```python
from build123d import *

# Parameters (mm, degrees)
F0_R     = 3.1
F0_R_2   = 1.6
F1_DEPTH = 5


with BuildPart() as f1:
    # F0 (on Front) → F1 (new body)
    with BuildSketch(Plane.XZ):
        with BuildLine():
            Line((10.150758, 20), (-10.150758, 20))
            ThreePointArc((-10.150758, 20), (-12.064175, 20.380602), (-13.686292, 21.464466))
            Line((-13.686292, 21.464466), (-61.509049, 69.287223))
            Line((-61.509049, 69.287223), (-67.386104, 73.484299))
            ThreePointArc((-67.386104, 73.484299), (-72.699434, 72.699434), (-73.484299, 67.386104))
            Line((-73.484299, 67.386104), (-69.287223, 61.509049))
            Line((-69.287223, 61.509049), (-21.464466, 13.686292))
            ThreePointArc((-21.464466, 13.686292), (-20.380602, 12.064175), (-20, 10.150758))
            Line((-20, 10.150758), (-20, -10.150758))
            ThreePointArc((-20, -10.150758), (-20.380602, -12.064175), (-21.464466, -13.686292))
            Line((-21.464466, -13.686292), (-69.287223, -61.509049))
            Line((-69.287223, -61.509049), (-73.484299, -67.386104))
            ThreePointArc((-73.484299, -67.386104), (-72.699434, -72.699434), (-67.386104, -73.484299))
            Line((-67.386104, -73.484299), (-61.509049, -69.287223))
            Line((-61.509049, -69.287223), (-13.686292, -21.464466))
            ThreePointArc((-13.686292, -21.464466), (-12.064175, -20.380602), (-10.150758, -20))
            Line((-10.150758, -20), (10.150758, -20))
            ThreePointArc((10.150758, -20), (12.064175, -20.380602), (13.686292, -21.464466))
            Line((13.686292, -21.464466), (61.509049, -69.287223))
            Line((61.509049, -69.287223), (67.386104, -73.484299))
            ThreePointArc((67.386104, -73.484299), (72.699434, -72.699434), (73.484299, -67.386104))
            Line((73.484299, -67.386104), (69.287223, -61.509049))
            Line((69.287223, -61.509049), (21.464466, -13.686292))
            ThreePointArc((21.464466, -13.686292), (20.380602, -12.064175), (20, -10.150758))
            Line((20, -10.150758), (20, 10.150758))
            ThreePointArc((20, 10.150758), (20.380602, 12.064175), (21.464466, 13.686292))
            Line((21.464466, 13.686292), (69.287223, 61.509049))
            Line((69.287223, 61.509049), (73.484299, 67.386104))
            ThreePointArc((73.484299, 67.386104), (72.699434, 72.699434), (67.386104, 73.484299))
            Line((67.386104, 73.484299), (61.509049, 69.287223))
            Line((61.509049, 69.287223), (13.686292, 21.464466))
            ThreePointArc((13.686292, 21.464466), (12.064175, 20.380602), (10.150758, 20))
        make_face()
        with BuildLine():
            ThreePointArc((-62.586144, -64.848885), (-64.848885, -64.848885), (-64.848885, -62.586144))
            Line((-64.848885, -62.586144), (-63.788225, -61.525483))
            ThreePointArc((-63.788225, -61.525483), (-61.525483, -61.525483), (-61.525483, -63.788225))
            Line((-61.525483, -63.788225), (-62.586144, -64.848885))
        make_face(mode=Mode.SUBTRACT)
        with Locations((-57, -57)):
            Circle(F0_R, mode=Mode.SUBTRACT)
        with BuildLine():
            ThreePointArc((-51.413856, -49.151115), (-49.151115, -49.151115), (-49.151115, -51.413856))
            Line((-49.151115, -51.413856), (-50.211775, -52.474517))
            ThreePointArc((-50.211775, -52.474517), (-52.474517, -52.474517), (-52.474517, -50.211775))
            Line((-52.474517, -50.211775), (-51.413856, -49.151115))
        make_face(mode=Mode.SUBTRACT)
        with Locations((-20.584001, -20.584001)):
            Circle(F0_R_2, mode=Mode.SUBTRACT)
        with Locations((-15.5, -15.5)):
            Circle(F0_R_2, mode=Mode.SUBTRACT)
        with BuildLine():
            ThreePointArc((64.848885, -62.586144), (64.848885, -64.848885), (62.586144, -64.848885))
            Line((62.586144, -64.848885), (61.525483, -63.788225))
            ThreePointArc((61.525483, -63.788225), (61.525483, -61.525483), (63.788225, -61.525483))
            Line((63.788225, -61.525483), (64.848885, -62.586144))
        make_face(mode=Mode.SUBTRACT)
        with Locations((57, -57)):
            Circle(F0_R, mode=Mode.SUBTRACT)
        with BuildLine():
            ThreePointArc((49.151115, -51.413856), (49.151115, -49.151115), (51.413856, -49.151115))
            Line((51.413856, -49.151115), (52.474517, -50.211775))
            ThreePointArc((52.474517, -50.211775), (52.474517, -52.474517), (50.211775, -52.474517))
            Line((50.211775, -52.474517), (49.151115, -51.413856))
        make_face(mode=Mode.SUBTRACT)
        with Locations((20.584001, -20.584001)):
            Circle(F0_R_2, mode=Mode.SUBTRACT)
        with Locations((15.5, -15.5)):
            Circle(F0_R_2, mode=Mode.SUBTRACT)
        with BuildLine():
            ThreePointArc((-10.80108, 10.5), (-10.654634, 10.853553), (-10.30108, 11))
            Line((-10.30108, 11), (-8.80108, 11))
            ThreePointArc((-8.80108, 11), (-8.447527, 10.853553), (-8.30108, 10.5))
            Line((-8.30108, 10.5), (-8.30108, -10.5))
            ThreePointArc((-8.30108, -10.5), (-8.447527, -10.853553), (-8.80108, -11))
            Line((-8.80108, -11), (-10.30108, -11))
            ThreePointArc((-10.30108, -11), (-10.654634, -10.853553), (-10.80108, -10.5))
            Line((-10.80108, -10.5), (-10.80108, 10.5))
        make_face(mode=Mode.SUBTRACT)
        with Locations((-15.5, 15.5)):
            Circle(F0_R_2, mode=Mode.SUBTRACT)
        with Locations((-20.584001, 20.584001)):
            Circle(F0_R_2, mode=Mode.SUBTRACT)
        with BuildLine():
            Line((-50.211775, 52.474517), (-49.151115, 51.413856))
            ThreePointArc((-49.151115, 51.413856), (-49.151115, 49.151115), (-51.413856, 49.151115))
            Line((-51.413856, 49.151115), (-52.474517, 50.211775))
            ThreePointArc((-52.474517, 50.211775), (-52.474517, 52.474517), (-50.211775, 52.474517))
        make_face(mode=Mode.SUBTRACT)
        with Locations((-57, 57)):
            Circle(F0_R, mode=Mode.SUBTRACT)
        with BuildLine():
            ThreePointArc((-64.848885, 62.586144), (-64.848885, 64.848885), (-62.586144, 64.848885))
            Line((-62.586144, 64.848885), (-61.525483, 63.788225))
            ThreePointArc((-61.525483, 63.788225), (-61.525483, 61.525483), (-63.788225, 61.525483))
            Line((-63.788225, 61.525483), (-64.848885, 62.586144))
        make_face(mode=Mode.SUBTRACT)
        with BuildLine():
            Line((10.80108, 10.5), (10.80108, -10.5))
            ThreePointArc((10.80108, -10.5), (10.654634, -10.853553), (10.30108, -11))
            Line((10.30108, -11), (8.80108, -11))
            ThreePointArc((8.80108, -11), (8.447527, -10.853553), (8.30108, -10.5))
            Line((8.30108, -10.5), (8.30108, 10.5))
            ThreePointArc((8.30108, 10.5), (8.447527, 10.853553), (8.80108, 11))
            Line((8.80108, 11), (10.30108, 11))
            ThreePointArc((10.30108, 11), (10.654634, 10.853553), (10.80108, 10.5))
        make_face(mode=Mode.SUBTRACT)
        with Locations((15.5, 15.5)):
            Circle(F0_R_2, mode=Mode.SUBTRACT)
        with Locations((20.584001, 20.584001)):
            Circle(F0_R_2, mode=Mode.SUBTRACT)
        with BuildLine():
            Line((52.474517, 50.211775), (51.413856, 49.151115))
            ThreePointArc((51.413856, 49.151115), (49.151115, 49.151115), (49.151115, 51.413856))
            Line((49.151115, 51.413856), (50.211775, 52.474517))
            ThreePointArc((50.211775, 52.474517), (52.474517, 52.474517), (52.474517, 50.211775))
        make_face(mode=Mode.SUBTRACT)
        with Locations((57, 57)):
            Circle(F0_R, mode=Mode.SUBTRACT)
        with BuildLine():
            ThreePointArc((62.586144, 64.848885), (64.848885, 64.848885), (64.848885, 62.586144))
            Line((64.848885, 62.586144), (63.788225, 61.525483))
            ThreePointArc((63.788225, 61.525483), (61.525483, 61.525483), (61.525483, 63.788225))
            Line((61.525483, 63.788225), (62.586144, 64.848885))
        make_face(mode=Mode.SUBTRACT)
    extrude(amount=F1_DEPTH)


solid = f1.part
```
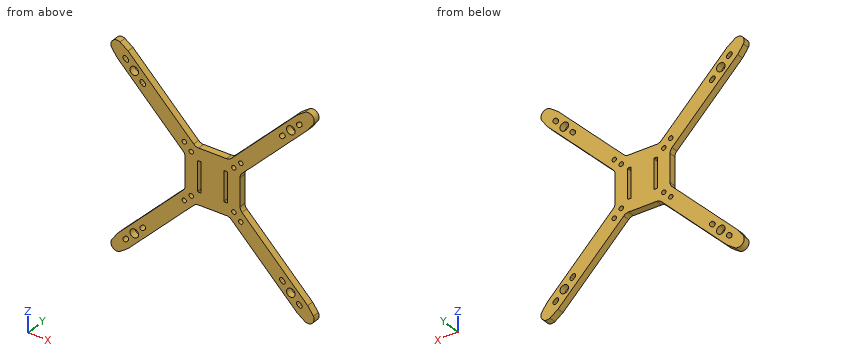
Work out the finished part from the listing and answer in its coordinate system (mm). Round coordinates to 2 decimals unless told otherwise and drop trailing zeros. Order: outer loops, then holes, each group sorted by start corner. A loop starts at its lowest first (then second) coordinate and runs counter-clockwise, first axis right, second up.
Q1. A cutting plane is placed at B-B, the plane x = 57. Determine the outline of the cut face in (y, z), then the cut area to 3 significant figures.
Solution:
outline: (-5, -64.78) - (0, -64.78) - (0, -60.1) - (-5, -60.1) - close; (-5, -53.9) - (0, -53.9) - (0, -49.22) - (-5, -49.22) - close; (-5, 49.22) - (0, 49.22) - (0, 53.9) - (-5, 53.9) - close; (-5, 60.1) - (0, 60.1) - (0, 64.78) - (-5, 64.78) - close
area: 93.6 mm2
Q2. A cutting plane is placed at A-A, the plane z = 6. Determine the outline of the cut face in (x, y), then the cut area to 3 significant figures.
Solution:
outline: (-20, -5) - (-10.8, -5) - (-10.8, 0) - (-20, 0) - close; (-8.3, -5) - (8.3, -5) - (8.3, 0) - (-8.3, 0) - close; (10.8, -5) - (20, -5) - (20, 0) - (10.8, 0) - close
area: 175 mm2
Q3. Find the intervals of material crossed by line 1 along X through (y, z) = (-3.95, 54.5); line 2 along Z through (x, y) = (63, -3.5); line 3 along X through (y, z) = (-1.45, -7), in increasing order.
Solution:
line 1: x = -62.28 to -58.83, -55.17 to -46.72, 46.72 to 55.17, 58.83 to 62.28
line 2: z = -70.35 to -65.15, -61.09 to -55.22, 55.22 to 61.09, 65.15 to 70.35
line 3: x = -20 to -10.8, -8.3 to 8.3, 10.8 to 20
Q4. A cutting plane is placed at D-D, the plane x = -4. Determine the outline of the cut face in (y, z).
Solution:
outline: (-5, -20) - (0, -20) - (0, 20) - (-5, 20) - close
Q5. Given pin 1 Ø1.5 at (y, z) = (-3, -1.5) entering from +X; pin 2 Ø2.5 at (y, z) = (-2.5, -3) entering from -X; pin 3 Ø3 at (x, y) = (40, -1) entering from +Z; pin 4 Ø4 at (x, z) = (20.58, -20.58) entering from -Y, each flat-ended and moving along its own axis, determine where each tip first touches the part or whether it passes through.
Solution:
pin 1: stops at x = 20
pin 2: stops at x = -20
pin 3: stops at z = 49.28
pin 4: stops at y = -5
Q6. A cutting plane is placed at C-C, the plane z = -57. Determine the outline of the cut face in (x, y).
Solution:
outline: (-64.78, -5) - (-60.1, -5) - (-60.1, 0) - (-64.78, 0) - close; (-53.9, -5) - (-49.22, -5) - (-49.22, 0) - (-53.9, 0) - close; (49.22, -5) - (53.9, -5) - (53.9, 0) - (49.22, 0) - close; (60.1, -5) - (64.78, -5) - (64.78, 0) - (60.1, 0) - close
